For this review, take the finished solid that the model builds, in its own axes (mm). Give positions to 0.01 mm unless a question says otherwise; leave off trailing zeros. Write each loop counter-clockwise with the first axis right and the second up, starting at its lowest first coordinate (ties: lowest second). Pieces come first, ordered by that corner, then holes.
1) We need section A-A on x = 193. Give the boundary of the cut face in (y, z), and give its area (3 significant figures).
2) For P1, Ø11.5, axis at x = 93, z = -78, coming from the +Y side, flat-tipped, find the tip position at first contact; note if it passes through.
3) Draft analysis for pull direction X (two halves, no side actions). For faces 1 (the face through (-94.915, 1.479, -73.381)), 2 (the face through (189, 1, 75)), 3 (the face through (244.99, 1.48, -90.15)), 4 (the face through (3, 3, -1)), state which applies: pulls with the +X half, pulls with the -X half, needs draft (parallel to the pull), parting line crosses it, or undercut.
4) We need section C-C on z = -38. Give the boundary of the cut face in (x, y), and give its area (3 significant figures).
5) We need section B-B on z = -78. Give the boundary of the cut face in (x, y), and give its area (3 significant figures).
6) Wall thickness on line 1 along X through (y, z) = (1.8, -78); line 2 along Z through (x, y) = (92.5, 0.6); line 3 along X through (y, z) = (0.8, 39.5): over which ranges is each line inside the solid? List them lowest first.
from build123d import *

# Parameters (mm, degrees)
SKETCH1_R           = 5
BOSS_EXTRUDE1_DEPTH = 3


with BuildPart() as part:
    # Sketch1 → Boss-Extrude1 (new body)
    with BuildSketch(Plane(origin=(0, 0, 0), x_dir=(1, 0, 0), z_dir=(0, 1, 0))):
        with BuildLine():
            Line((-238, 93), (238, 93))
            ThreePointArc((238, 93), (245.071067812, 90.071067812), (248, 83))
            Line((248, 83), (248, -83))
            ThreePointArc((248, -83), (245.071067812, -90.071067812), (238, -93))
            Line((238, -93), (-238, -93))
            ThreePointArc((-238, -93), (-245.071067812, -90.071067812), (-248, -83))
            Line((-248, -83), (-248, 83))
            ThreePointArc((-248, 83), (-245.071067812, 90.071067812), (-238, 93))
        make_face()
        with Locations(Location((-193, 78, 0), (0, 0, 270))):
            Circle(SKETCH1_R, mode=Mode.SUBTRACT)
        with Locations(Location((-93, 78, 0), (0, 0, 270))):
            Circle(SKETCH1_R, mode=Mode.SUBTRACT)
        with Locations(Location((0, 78, 0), (0, 0, 270))):
            Circle(SKETCH1_R, mode=Mode.SUBTRACT)
        with Locations(Location((-233, 38, 0), (0, 0, 270))):
            Circle(SKETCH1_R, mode=Mode.SUBTRACT)
        with Locations(Location((93, 78, 0), (0, 0, 270))):
            Circle(SKETCH1_R, mode=Mode.SUBTRACT)
        with Locations(Location((193, 78, 0), (0, 0, 270))):
            Circle(SKETCH1_R, mode=Mode.SUBTRACT)
        with Locations(Location((233, 38, 0), (0, 0, 270))):
            Circle(SKETCH1_R, mode=Mode.SUBTRACT)
        with Locations(Location((233, -38, 0), (0, 0, 90))):
            Circle(SKETCH1_R, mode=Mode.SUBTRACT)
        with Locations(Location((193, -78, 0), (0, 0, 90))):
            Circle(SKETCH1_R, mode=Mode.SUBTRACT)
        with Locations(Location((93, -78, 0), (0, 0, 90))):
            Circle(SKETCH1_R, mode=Mode.SUBTRACT)
        with Locations(Location((0, -78, 0), (0, 0, 90))):
            Circle(SKETCH1_R, mode=Mode.SUBTRACT)
        with Locations(Location((-93, -78, 0), (0, 0, 90))):
            Circle(SKETCH1_R, mode=Mode.SUBTRACT)
        with Locations(Location((-193, -78, 0), (0, 0, 90))):
            Circle(SKETCH1_R, mode=Mode.SUBTRACT)
        with Locations(Location((-233, -38, 0), (0, 0, 90))):
            Circle(SKETCH1_R, mode=Mode.SUBTRACT)
    extrude(amount=BOSS_EXTRUDE1_DEPTH)


solid = part.part
Results list:
1. outline: (0, -93) - (3, -93) - (3, -83) - (0, -83) - close; (0, -73) - (3, -73) - (3, 73) - (0, 73) - close; (0, 83) - (3, 83) - (3, 93) - (0, 93) - close
1. area: 498 mm2
2. P1: stops at y = 3
3. face 1: undercut
3. face 2: undercut
3. face 3: pulls with the +X half
3. face 4: needs draft
4. outline: (-248, 0) - (-238, 0) - (-238, 3) - (-248, 3) - close; (-228, 0) - (228, 0) - (228, 3) - (-228, 3) - close; (238, 0) - (248, 0) - (248, 3) - (238, 3) - close
4. area: 1,430 mm2
5. outline: (-248, 0) - (-198, 0) - (-198, 3) - (-248, 3) - close; (-188, 0) - (-98, 0) - (-98, 3) - (-188, 3) - close; (-88, 0) - (-5, 0) - (-5, 3) - (-88, 3) - close; (5, 0) - (88, 0) - (88, 3) - (5, 3) - close; (98, 0) - (188, 0) - (188, 3) - (98, 3) - close; (198, 0) - (248, 0) - (248, 3) - (198, 3) - close
5. area: 1,340 mm2
6. line 1: x = -248 to -198, -188 to -98, -88 to -5, 5 to 88, 98 to 188, 198 to 248
6. line 2: z = -93 to -82.97, -73.03 to 73.03, 82.97 to 93
6. line 3: x = -248 to -237.77, -228.23 to 228.23, 237.77 to 248
